Here's how the part is built. I have some questions about the finished solid (model axes, mm). Face numbers are marked on the shaded views. Round coordinates to 2 decimals unless told otherwise and drop trailing zeros. Loops run counter-clockwise (first coordinate to the right, second up) from the corner with the lowest first, then second, coordinate; pieces in that order, holes last. Notation, with made-up numbers: (76, -17) -> (102, -17) arc R25 ccw to (102, 0) -> close; hole circle Ø3 at (81, 64). An arc over 180 degrees is marked (long way). Use one line per item in the form item = value. Start each with the question number.
Item 1: If we section it at A-A (z = 19.5): Write out the boundary of the cut face in (x, y).
Item 2: Thinking about a two-plate mould opening in X: for the marked faces 1, 2, 3 and 4, which applies, released by +X, released by -X, zero draft, split by the parting line, or undercut?
Item 3: I'm going to push flat-ended pins straight in: pin 1 Ø2 at (x, y) = (-66.5, -51) entering from -Z; pin 2 Ø1.5 at (y, z) = (42.5, 44.5) entering from +X; pin 3 Ø10 at (y, z) = (26, 43) entering from +X. Where does each tip first touch, or does it pass through?
Item 4: If I drill on L1, parallel to Y at x = 0, z = -2.9; L2, parallel to Y at x = 0, z = 20.5; L3, parallel to Z at x = -16.5, y = 63, over which ranges is the centre line in solid material (lowest first)? Write a range as [from, to].
```python
from build123d import *

# Parameters (mm, degrees)
SKETCH1_R           = 89.45
SKETCH1_R_2         = 76.75
BOSS_EXTRUDE1_DEPTH = 33
BOSS_EXTRUDE2_START = 5
SKETCH2_R           = 89.45
SKETCH2_R_2         = 85
BOSS_EXTRUDE2_DEPTH = 5
SKETCH3_R           = 89.45
BOSS_EXTRUDE3_DEPTH = 20
CHAMFER1_SIZE       = 15
CHAMFER2_SIZE       = 5
CHAMFER2_SIZE2      = 1.819851171
FILLET1_R           = 10
FILLET2_R           = 2
FILLET3_R           = 5


with BuildPart() as part:
    # Sketch1 → Boss-Extrude1 (new body)
    with BuildSketch(Plane.XY):
        Circle(SKETCH1_R)
        Circle(SKETCH1_R_2, mode=Mode.SUBTRACT)
    extrude(amount=BOSS_EXTRUDE1_DEPTH)

    # Sketch2 → Boss-Extrude2 (add)
    with BuildSketch(Plane(origin=(0, 0, 0), x_dir=(-1, 0, 0), z_dir=(0, 0, -1)).offset(BOSS_EXTRUDE2_START)):
        Circle(SKETCH2_R)
        Circle(SKETCH2_R_2, mode=Mode.SUBTRACT)
    extrude(amount=-BOSS_EXTRUDE2_DEPTH)

    # Sketch3 → Boss-Extrude3 (add)
    with BuildSketch(Plane.XY.offset(33)):
        with Locations(Location((0, 0, 0), (0, 0, 180))):
            Circle(SKETCH3_R)
    extrude(amount=BOSS_EXTRUDE3_DEPTH)

    # Chamfer1
    chamfer1_edges = [part.edges().sort_by_distance(p)[0] for p in [
        (89.45, 0, 53),
    ]]
    chamfer(chamfer1_edges, length=CHAMFER1_SIZE)

    # Chamfer2
    chamfer2_edges = [part.edges().sort_by_distance(p)[0] for p in [
        (-76.75, 0, 0),
    ]]
    chamfer2_side = [part.faces().sort_by_distance(p)[0] for p in [
        (-76.75, 0, 16.5),
    ]]
    chamfer(chamfer2_edges, length=CHAMFER2_SIZE, length2=CHAMFER2_SIZE2, reference=chamfer2_side[0])

    # Fillet1
    fillet1_edges = [part.edges().sort_by_distance(p)[0] for p in [
        (-76.75, 0, 5),
    ]]
    fillet(fillet1_edges, radius=FILLET1_R)

    # Fillet2
    fillet2_edges = [part.edges().sort_by_distance(p)[0] for p in [
        (-78.569851171, 0, 0),
    ]]
    fillet(fillet2_edges, radius=FILLET2_R)

    # Fillet3
    fillet3_edges = [part.edges().sort_by_distance(p)[0] for p in [
        (-76.75, 0, 33),
    ]]
    fillet(fillet3_edges, radius=FILLET3_R)


solid = part.part
```
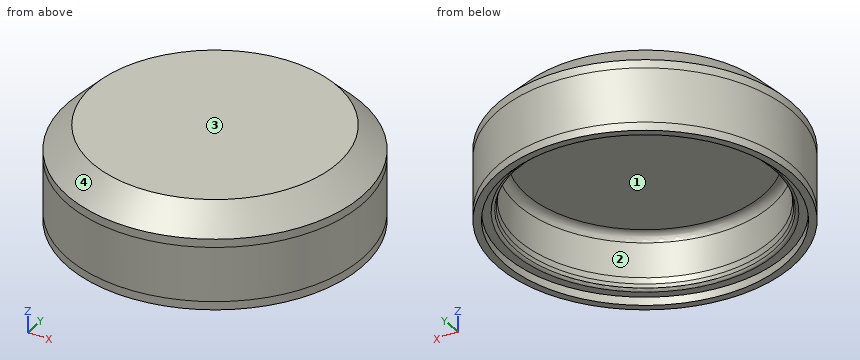
Values found:
q1.outline = circle Ø178.9 at (0, 0); hole circle Ø153.5 at (0, 0)
q2.face_1 = undercut
q2.face_2 = undercut
q2.face_3 = zero draft
q2.face_4 = split by the parting line
q3.pin_1 = 0
q3.pin_2 = 72.21
q3.pin_3 = 85.79
q4.L1 = [-89.45, -85], [85, 89.45]
q4.L2 = [-89.45, -76.75], [76.75, 89.45]
q4.L3 = [33, 53]
